Input: part model. Units: mm. Frame: model coordinates. A direction names the side the tool comes from. Coordinates: 2 decimals unless noted, no trailing zeros. Write each loop counter-clockwise with the first axis right and the second up, starting at its lowest first coordinate (ties: lowest second). Pieces come first, ordered by that corner, then holes.
from build123d import *

# Parameters (mm, degrees)
SKETCH_1_W                = 78
SKETCH_1_H                = 15
EXTRUDE_1_DEPTH           = 3
SKETCH_3_R                = 1.5
CUT_EXTRUDE_1_DEPTH       = 3
SKETCH_4_R                = 6
EXTRUDE_2_DEPTH           = 18
SKETCH_5_R                = 4.5
CUT_EXTRUDE_2_DEPTH       = 21
F_2_0MM_2_D               = 3
F_2_0MM_2_DEPTH           = 4.5
F_2_0MM_2_TIP             = 1.5
F_2_0MM_2_ON_FACE_2_D     = 3
F_2_0MM_2_ON_FACE_2_DEPTH = 4.5
F_2_0MM_2_ON_FACE_2_TIP   = 1.5
SKETCH_10_W               = 6
SKETCH_10_H               = 10
CUT_EXTRUDE_3_DEPTH       = 7
SKETCH_13_W               = 19.835687411
SKETCH_13_H               = 21.610205193
CUT_EXTRUDE_4_DEPTH       = 20
SKETCH_14_W               = 11.523038103
SKETCH_14_H               = 10.49031299
EXTRUDE_3_DEPTH           = 3
SKETCH_18_W               = 78
SKETCH_18_H               = 8
EXTRUDE_4_DEPTH           = 3
SKETCH_19_W               = 36.767904102
SKETCH_19_H               = 2.5
EXTRUDE_5_DEPTH           = 12.5
SKETCH_23_R               = 1.65
CUT_EXTRUDE_6_DEPTH       = 12.5
SKETCH_25_W               = 4.236607592
SKETCH_25_H               = 5.36409187
EXTRUDE_7_DEPTH           = 2.5
SKETCH_26_R               = 1.6
CUT_EXTRUDE_7_DEPTH       = 2.5


with BuildPart() as part:
    # 草图1 → 凸台-拉伸1 (new body)
    with BuildSketch(Plane(origin=(0, 0, 0), x_dir=(1, 0, 0), z_dir=(0, 1, 0))):
        Rectangle(SKETCH_1_W, SKETCH_1_H)
    extrude(amount=EXTRUDE_1_DEPTH)

    # 草图3 → 切除-拉伸1 (cut)
    with BuildSketch(Plane(origin=(0, 3, 0), x_dir=(1, 0, 0), z_dir=(0, 1, 0))):
        with Locations(Location((-34.76, -1.72, 0), (0, 0, 270))):
            Circle(SKETCH_3_R)
        with Locations(Location((-24.35, 4.1, 0), (0, 0, 270))):
            Circle(SKETCH_3_R)
        with Locations(Location((31.56, 4.221692081, 0), (0, 0, 270))):
            Circle(SKETCH_3_R)
        with Locations(Location((7.56, 4.221692081, 0), (0, 0, 270))):
            Circle(SKETCH_3_R)
    extrude(amount=-CUT_EXTRUDE_1_DEPTH, mode=Mode.SUBTRACT)

    # 草图4 → 凸台-拉伸2 (add)
    with BuildSketch(Plane(origin=(0, 3, 0), x_dir=(1, 0, 0), z_dir=(0, 1, 0))):
        with Locations(Location((-3, -1.234165229, 0), (0, 0, 270))):
            Circle(SKETCH_4_R)
    extrude(amount=EXTRUDE_2_DEPTH)

    # 草图5 → 切除-拉伸2 (cut)
    with BuildSketch(Plane(origin=(0, 21, 0), x_dir=(1, 0, 0), z_dir=(0, 1, 0))):
        with Locations(Location((-3, -1.234165229, 0), (0, 0, 270))):
            Circle(SKETCH_5_R)
    extrude(amount=-CUT_EXTRUDE_2_DEPTH, mode=Mode.SUBTRACT)

    # Ø2.0mm 暗销孔2
    with Locations(Plane(origin=(-7.901331048, 17.342107422, 4.694938836), x_dir=(-0.576795601176, 0, -0.816888507977), z_dir=(-0.816888507977, 0, 0.576795601176))):
        with Locations((0, 0)):
            Hole(F_2_0MM_2_D / 2, depth=F_2_0MM_2_DEPTH)
            with Locations((0, 0, -(F_2_0MM_2_DEPTH + F_2_0MM_2_TIP / 2))):  # 90° drill point
                Cone(0, F_2_0MM_2_D / 2, F_2_0MM_2_TIP, mode=Mode.SUBTRACT)

    # Ø2.0mm 暗销孔2 on face 2
    with Locations(Plane(origin=(1.071764877, 17.164817099, 5.641061052), x_dir=(0.734483043181, 0, -0.678627039897), z_dir=(0.678627039897, 0, 0.734483043181))):
        with Locations((0, 0)):
            Hole(F_2_0MM_2_ON_FACE_2_D / 2, depth=F_2_0MM_2_ON_FACE_2_DEPTH)
            with Locations((0, 0, -(F_2_0MM_2_ON_FACE_2_DEPTH + F_2_0MM_2_ON_FACE_2_TIP / 2))):  # 90° drill point
                Cone(0, F_2_0MM_2_ON_FACE_2_D / 2, F_2_0MM_2_ON_FACE_2_TIP, mode=Mode.SUBTRACT)

    # 草图10 → 切除-拉伸3 (cut)
    with BuildSketch(Plane(origin=(0, 0, -7.5), x_dir=(-1, 0, 0), z_dir=(0, 0, -1))):
        with Locations((3, 8)):
            Rectangle(SKETCH_10_W, SKETCH_10_H)
    extrude(amount=-CUT_EXTRUDE_3_DEPTH, mode=Mode.SUBTRACT)

    # 草图13 → 切除-拉伸4 (cut)
    with BuildSketch(Plane(origin=(0, 0, -7.5), x_dir=(-1, 0, 0), z_dir=(0, 0, -1))):
        with Locations((3.314421038, 13.805102597)):
            Rectangle(SKETCH_13_W, SKETCH_13_H)
    extrude(amount=-CUT_EXTRUDE_4_DEPTH, mode=Mode.SUBTRACT)

    # 草图14 → 凸台-拉伸3 (add)
    with BuildSketch(Plane(origin=(0, 3, 0), x_dir=(1, 0, 0), z_dir=(0, 1, 0))):
        with Locations((-2.989467433, -1.263493391)):
            Rectangle(SKETCH_14_W, SKETCH_14_H)
    extrude(amount=-EXTRUDE_3_DEPTH)

    # 草图18 → 凸台-拉伸4 (add)
    with BuildSketch(Plane.XZ):
        with Locations((0, 11.5)):
            Rectangle(SKETCH_18_W, SKETCH_18_H)
    extrude(amount=-EXTRUDE_4_DEPTH)

    # 草图19 → 凸台-拉伸5 (add)
    with BuildSketch(Plane.XZ):
        with Locations((0.839237194, 14.25)):
            Rectangle(SKETCH_19_W, SKETCH_19_H)
    extrude(amount=EXTRUDE_5_DEPTH)

    # 草图23 → 切除-拉伸6 (cut)
    with BuildSketch(Plane(origin=(0, 0, 13), x_dir=(-1, 0, 0), z_dir=(0, 0, -1))):
        with Locations((-8.603189245, -6.05592298)):
            Circle(SKETCH_23_R)
        with Locations((2.596810755, -6.05592298)):
            Circle(SKETCH_23_R)
    extrude(amount=-CUT_EXTRUDE_6_DEPTH, mode=Mode.SUBTRACT)

    # 草图25 → 凸台-拉伸7 (add)
    with BuildSketch(Plane(origin=(0, 0, 13), x_dir=(-1, 0, 0), z_dir=(0, 0, -1))):
        with Locations((2.330668631, -6.426480946)):
            Rectangle(SKETCH_25_W, SKETCH_25_H)
    extrude(amount=-EXTRUDE_7_DEPTH)

    # 草图26 → 切除-拉伸7 (cut)
    with BuildSketch(Plane(origin=(0, 0, 13), x_dir=(-1, 0, 0), z_dir=(0, 0, -1))):
        with Locations((4.196810755, -6.05592298)):
            Circle(SKETCH_26_R)
    extrude(amount=-CUT_EXTRUDE_7_DEPTH, mode=Mode.SUBTRACT)


solid = part.part
Item 1: Pin query (flat end, axial travel): pin 1 Ø3 at (y, z) = (-8.5, 14.5) entering from -X; pin 2 Ø1.2 at (y, z) = (-8, 14) entering from +X; pin 3 Ø4 at (x, y) = (8.6, -6.06) entering from -Z. Return the tip coordinate at first contact, or that it passes through.
Item 2: Section query C-C, the plane z = -4.1. Return loops of the section in (x, y), then the cut area to 3 significant figures.
Item 3: Section query A-A, the plane z = 1.72. Return loops of the section in (x, y), then the cut area to 3 significant figures.
Item 4: Section query B-B, the plane x = -34.76. Return loops of the section in (y, z).
Item 5: Access query for faces 4 (the face through (1, -6, 13)), 5 (the face through (-1, 3, 4)), 6 (the face through (19.223, -6, 14)). Directions: +Z, -Z, +X, -X, +Y, -Y. A direction counts if a zero-diameter tool reaches every point of the face in a straight line with its end or side. Return the directions, or none.
Item 6: Section query D-D, the plane x = 2. Return loops of the section in (y, z), then the cut area to 3 significant figures.
Item 7: Pull-direction query (Z, two-part tool) for faces 1 (the face through (33.047, 1.521, -4.417)), 2 (the face through (-17.545, -6, 14)), 3 (the face through (-1, -3, 15.5)); classes: released by +Z, released by -Z, zero draft, split by the parting line, or undercut.
Item 8: Material intervals for line 1 (Y direction, x = -33, z = 6.25); line 2 (Z direction, x = 15, y = -4); line 3 (X direction, y = 2, z = 1.5), sorted ascending.
The answers:
1. pin 1: stops at x = -17.54
1. pin 2: stops at x = 19.22
1. pin 3: stops at z = 13
2. outline: (-39, 0) - (-25.85, 0) - (-25.85, 3) - (-39, 3) - close; (-22.85, 0) - (6.06, 0) - (6.06, 3) - (-22.85, 3) - close; (9.06, 0) - (30.06, 0) - (30.06, 3) - (9.06, 3) - close; (33.06, 0) - (39, 0) - (39, 3) - (33.06, 3) - close
2. area: 207 mm2
3. outline: (-39, 0) - (-36.26, 0) - (-36.26, 3) - (-39, 3) - close; (-33.26, 0) - (39, 0) - (39, 3) - (-33.26, 3) - close
3. area: 225 mm2
4. outline: (0, -7.5) - (3, -7.5) - (3, 0.22) - (0, 0.22) - close; (0, 3.22) - (3, 3.22) - (3, 15.5) - (0, 15.5) - close
5. face 4: -Z, +X, -X, -Y
5. face 5: +Z, -Z, +X, -X, +Y
5. face 6: +Z, -Z, +X, -Y
6. outline: (-12.5, 13) - (0, 13) - (0, -7.5) - (3, -7.5) - (3, 15.5) - (-12.5, 15.5) - close
6. area: 100 mm2
7. face 1: undercut
7. face 2: zero draft
7. face 3: released by +Z
8. line 1: y = 0 to 3
8. line 2: z = 13 to 15.5
8. line 3: x = -39 to -36.24, -33.28 to 39
